from build123d import *

# Parameters (mm, degrees)
CUT_EXTRUDE1_DEPTH      = 37.041642582
CUT_EXTRUDE2_DEPTH      = 37.041642582
CUT_EXTRUDE2_DEPTH_BACK = 37.041642582
SKETCH4_R               = 1
SKETCH6_R               = 2.25
CUT_EXTRUDE3_DEPTH      = 37.04164274


with BuildPart() as part:
    # Sketch2 → Revolve1 (revolve)
    with BuildSketch(Plane(origin=(0, 0, 0), x_dir=(1, 0, 0), z_dir=(0, 1, 0))):
        with BuildLine():
            Line((25, 6), (25, 7))
            Line((25, 7), (0, 7))
            Line((0, 7), (0, 0))
            Line((0, 0), (25, 0))
            Line((25, 0), (25, 1))
            ThreePointArc((25, 1), (22.5, 3.5), (25, 6))
        make_face()
    revolve(axis=Axis((0, 0, 0), (0, 0, -1)))

    # Sketch3 → Cut-Extrude1 (cut, through all)
    with BuildSketch(Plane.XY):
        with BuildLine():
            Line((-1.658312395, 2.5), (1.658312395, 2.5))
            ThreePointArc((1.658312395, 2.5), (0, -3), (-1.658312395, 2.5))
        make_face()
    extrude(amount=-CUT_EXTRUDE1_DEPTH, mode=Mode.SUBTRACT)

    # Sketch4 → Cut-Extrude2 (cut, two sides: drawn at the far end of the back side and taken through both)
    with BuildSketch(Plane(origin=(0, 0, 0), x_dir=(1, 0, 0), z_dir=(0, 1, 0)).offset(-CUT_EXTRUDE2_DEPTH_BACK)):
        with Locations(Location((0, 3.5, 0), (0, 0, 270))):
            Circle(SKETCH4_R)
    extrude(amount=CUT_EXTRUDE2_DEPTH + CUT_EXTRUDE2_DEPTH_BACK, mode=Mode.SUBTRACT)

    # Sketch6 → Cut-Extrude3 (cut, through all)
    with BuildSketch(Plane(origin=(0, 0, 0), x_dir=(1, 0, 0), z_dir=(0, 1, 0))):
        with Locations(Location((0, 3.5, 0), (0, 0, 270))):
            Circle(SKETCH6_R)
    extrude(amount=-CUT_EXTRUDE3_DEPTH, mode=Mode.SUBTRACT)


solid = part.part
Input: part model. Units: mm. Frame: model coordinates. A direction names the side the tool comes from. Coordinates: 2 decimals unless noted, no trailing zeros. Order: outer loops, then holes, each group sorted by start corner. A loop starts at its lowest first (then second) coordinate and runs counter-clockwise, first axis right, second up.
1. Access query for faces 4 (the cylindrical face through (0.676, -12.794, -1.354)), 5 (the cylindrical face through (2.764, -1.166, -3.451)). Directions: +Z, -Z, +X, -X, +Y, -Y. A direction counts if a zero-diameter tool reaches every point of the face in a straight line with its end or side. Return the directions, or none.
Checked values:
face 4: -Y
face 5: +Z, -Z
2. Cut plane B-B, the plane y = 0. Return loops of the section in (x, z).
Checked values:
outline: (-25, -7) - (-3, -7) - (-3, 0) - (-25, 0) - (-25, -1) arc R2.5 cw to (-25, -6) - close; (3, -7) - (25, -7) - (25, -6) arc R2.5 cw to (25, -1) - (25, 0) - (3, 0) - close
3. Draft query along X for faces 1 (the cylindrical face through (23.846, -7.509, -0.507)), 2 (the flat face through (0, 5, 0)), 3 (the cylindrical face through (-0.6, 12.5, -4.3)). Return one class per face: +X half, -X half, draft (parallel to the pull), parting line (faces both ways), or undercut.
Checked values:
face 1: parting line
face 2: draft
face 3: undercut
4. Ray query, line 1 along Z through (x, y) = (0, -14.25); line 2 along Z through (x, y) = (0.5, 20.5); line 3 along X through (y, z) = (-4, -5). Return the intervals inside material, ascending.
Checked values:
line 1: z = -7 to -5.75, -1.25 to 0
line 2: z = -7 to -4.37, -2.63 to 0
line 3: x = -22.65 to -1.68, 1.68 to 22.65
5. Contact query for a flat-ended pin moving along its axis: P1, Ø2.5, axis at x = 0, z = -4, coming from the -Y side. Output: stop coordinate, or through.
Checked values:
P1: stops at y = 2.5
6. Cut plane A-A, the plane z = -3.5. Return loops of the section in (x, y), plus the area to 3 significant figures.
Checked values:
outline: (-2.25, -22.39) - (-2.25, -1.98) arc R3 cw to (-1.66, 2.5) - (-1, 2.5) - (-1, 22.48) arc R22.5 ccw to start; (1, 2.5) - (1.66, 2.5) arc R3 cw to (2.25, -1.98) - (2.25, -22.39) arc R22.5 ccw to (1, 22.48) - close
area: 1,430 mm2
